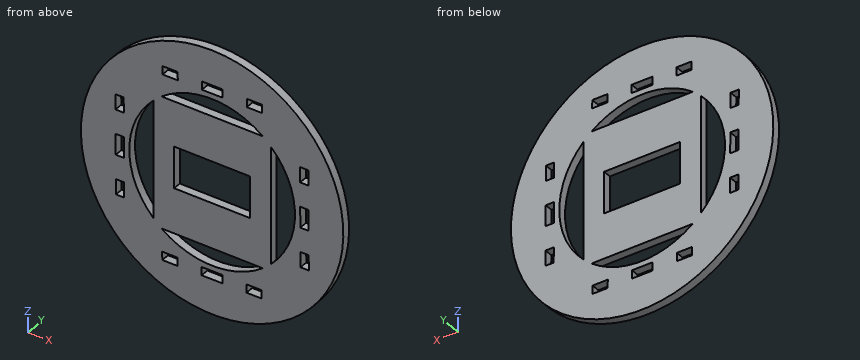
```python
from build123d import *

# Parameters (mm, degrees)
SKETCH1_R             = 95
BOSS_EXTRUDE1_DEPTH   = 6
SKETCH2_W             = 55
SKETCH2_H             = 30
CUT_EXTRUDE1_DEPTH    = 135.484199815
CAVITY1_START         = -69.821849164
CAVITY1_OUTLINE_W     = 15
CAVITY1_OUTLINE_H     = 6
CAVITY1_OUTLINE_W_2   = 11
CAVITY1_DEPTH         = 6
CAVITY1_START_2       = 63.821772898
CAVITY1_2_OUTLINE_W   = 11
CAVITY1_2_OUTLINE_H   = 6
CAVITY1_2_OUTLINE_W_2 = 15
CAVITY1_2_DEPTH       = 6
CAVITY1_START_3       = -7.051829773
CAVITY1_3_OUTLINE_W   = 6
CAVITY1_3_OUTLINE_H   = 6
CAVITY1_3_DEPTH       = 14.103659546
CAVITY1_START_4       = -35.551829773
CAVITY1_4_OUTLINE_W   = 6
CAVITY1_4_OUTLINE_H   = 6
CAVITY1_4_DEPTH       = 10.103659546
CAVITY1_START_5       = 25.448170227
CAVITY1_5_OUTLINE_W   = 6
CAVITY1_5_OUTLINE_H   = 6
CAVITY1_5_DEPTH       = 10.103659546
CAVITY1_START_6       = -36.448170227
CAVITY1_6_OUTLINE_W   = 6
CAVITY1_6_OUTLINE_H   = 6
CAVITY1_6_DEPTH       = 0.896340454
CAVITY1_START_7       = -25.448170227
CAVITY1_7_OUTLINE_W   = 6
CAVITY1_7_OUTLINE_H   = 6
CAVITY1_7_DEPTH       = 0.896340454
CAVITY1_START_8       = -7.948170227
CAVITY1_8_OUTLINE_W   = 6
CAVITY1_8_OUTLINE_H   = 6
CAVITY1_8_DEPTH       = 0.896340454
CAVITY1_START_9       = 7.051829773
CAVITY1_9_OUTLINE_W   = 6
CAVITY1_9_OUTLINE_H   = 6
CAVITY1_9_DEPTH       = 0.896340454
CAVITY1_START_10      = 24.551829773
CAVITY1_10_OUTLINE_W  = 6
CAVITY1_10_OUTLINE_H  = 6
CAVITY1_10_DEPTH      = 0.896340454
CAVITY1_START_11      = 35.551829773
CAVITY1_11_OUTLINE_W  = 6
CAVITY1_11_OUTLINE_H  = 6
CAVITY1_11_DEPTH      = 0.896340454


# Read off the part's stored shape, not the designer's step: Cavity1
with BuildPart() as part:
    # Sketch1 → Boss-Extrude1 (new body)
    with BuildSketch(Plane(origin=(0, 0, 0), x_dir=(1, 0, 0), z_dir=(0, 1, 0))):
        with Locations(Location((0, 0, 0), (0, 0, 270))):
            Circle(SKETCH1_R)
        with BuildLine():
            Line((-36.657195747, -47.5), (36.657195747, -47.5))
            ThreePointArc((36.657195747, -47.5), (0, -60), (-36.657195747, -47.5))
        make_face(mode=Mode.SUBTRACT)
        with BuildLine():
            Line((-42.5, 42.352685865), (-42.5, -42.352685865))
            ThreePointArc((-42.5, -42.352685865), (-60, 0), (-42.5, 42.352685865))
        make_face(mode=Mode.SUBTRACT)
        with BuildLine():
            Line((36.657195747, 47.5), (-36.657195747, 47.5))
            ThreePointArc((-36.657195747, 47.5), (0, 60), (36.657195747, 47.5))
        make_face(mode=Mode.SUBTRACT)
        with BuildLine():
            Line((42.5, -42.352685865), (42.5, 42.352685865))
            ThreePointArc((42.5, 42.352685865), (60, 0), (42.5, -42.352685865))
        make_face(mode=Mode.SUBTRACT)
    extrude(amount=BOSS_EXTRUDE1_DEPTH)

    # Sketch2 → Cut-Extrude1 (cut, through all)
    with BuildSketch(Plane(origin=(0, 6, 0), x_dir=(1, 0, 0), z_dir=(0, 1, 0))):
        Rectangle(SKETCH2_W, SKETCH2_H)
    extrude(amount=-CUT_EXTRUDE1_DEPTH, mode=Mode.SUBTRACT)

    # Cavity1 outline → Cavity1 (cut)
    with BuildSketch(Plane(origin=(0, 0, 0), x_dir=(0.9999872892756082, 0, 0.005041952719030872), z_dir=(0.005041952719030872, 0, -0.9999872892756083)).offset(CAVITY1_START)):
        with Locations((0.448170227, -3)):
            Rectangle(CAVITY1_OUTLINE_W, CAVITY1_OUTLINE_H)
        with Locations((30.948170227, -3)):
            Rectangle(CAVITY1_OUTLINE_W_2, CAVITY1_OUTLINE_H)
        with Locations((-30.051829773, -3)):
            Rectangle(CAVITY1_OUTLINE_W_2, CAVITY1_OUTLINE_H)
    extrude(amount=CAVITY1_DEPTH, mode=Mode.SUBTRACT)

    # Cavity1 2 outline → Cavity1 2 (cut)
    with BuildSketch(Plane(origin=(0, 0, 0), x_dir=(0.9999872892756082, 0, 0.005041952719030872), z_dir=(0.005041952719030872, 0, -0.9999872892756083)).offset(CAVITY1_START_2)):
        with Locations((30.051829773, -3)):
            Rectangle(CAVITY1_2_OUTLINE_W, CAVITY1_2_OUTLINE_H)
        with Locations((-0.448170227, -3)):
            Rectangle(CAVITY1_2_OUTLINE_W_2, CAVITY1_2_OUTLINE_H)
        with Locations((-30.948170227, -3)):
            Rectangle(CAVITY1_2_OUTLINE_W, CAVITY1_2_OUTLINE_H)
    extrude(amount=CAVITY1_2_DEPTH, mode=Mode.SUBTRACT)

    # Cavity1 3 outline → Cavity1 3 (cut)
    with BuildSketch(Plane(origin=(0, 0, 0), x_dir=(0.9999872892756082, 0, 0.005041952719030872), z_dir=(0.005041952719030872, 0, -0.9999872892756083)).offset(CAVITY1_START_3)):
        with Locations((66.821849164, -3)):
            Rectangle(CAVITY1_3_OUTLINE_W, CAVITY1_3_OUTLINE_H)
        with Locations((-66.821849164, -3)):
            Rectangle(CAVITY1_3_OUTLINE_W, CAVITY1_3_OUTLINE_H)
    extrude(amount=CAVITY1_3_DEPTH, mode=Mode.SUBTRACT)

    # Cavity1 4 outline → Cavity1 4 (cut)
    with BuildSketch(Plane(origin=(0, 0, 0), x_dir=(0.9999872892756082, 0, 0.005041952719030872), z_dir=(0.005041952719030872, 0, -0.9999872892756083)).offset(CAVITY1_START_4)):
        with Locations((66.821849164, -3)):
            Rectangle(CAVITY1_4_OUTLINE_W, CAVITY1_4_OUTLINE_H)
        with Locations((-66.821849164, -3)):
            Rectangle(CAVITY1_4_OUTLINE_W, CAVITY1_4_OUTLINE_H)
    extrude(amount=CAVITY1_4_DEPTH, mode=Mode.SUBTRACT)

    # Cavity1 5 outline → Cavity1 5 (cut)
    with BuildSketch(Plane(origin=(0, 0, 0), x_dir=(0.9999872892756082, 0, 0.005041952719030872), z_dir=(0.005041952719030872, 0, -0.9999872892756083)).offset(CAVITY1_START_5)):
        with Locations((66.821849164, -3)):
            Rectangle(CAVITY1_5_OUTLINE_W, CAVITY1_5_OUTLINE_H)
        with Locations((-66.821849164, -3)):
            Rectangle(CAVITY1_5_OUTLINE_W, CAVITY1_5_OUTLINE_H)
    extrude(amount=CAVITY1_5_DEPTH, mode=Mode.SUBTRACT)

    # Cavity1 6 outline → Cavity1 6 (cut)
    with BuildSketch(Plane(origin=(0, 0, 0), x_dir=(0.9999872892756082, 0, 0.005041952719030872), z_dir=(0.005041952719030872, 0, -0.9999872892756083)).offset(CAVITY1_START_6)):
        with Locations((-66.821849164, -3)):
            Rectangle(CAVITY1_6_OUTLINE_W, CAVITY1_6_OUTLINE_H)
    extrude(amount=CAVITY1_6_DEPTH, mode=Mode.SUBTRACT)

    # Cavity1 7 outline → Cavity1 7 (cut)
    with BuildSketch(Plane(origin=(0, 0, 0), x_dir=(0.9999872892756082, 0, 0.005041952719030872), z_dir=(0.005041952719030872, 0, -0.9999872892756083)).offset(CAVITY1_START_7)):
        with Locations((66.821849164, -3)):
            Rectangle(CAVITY1_7_OUTLINE_W, CAVITY1_7_OUTLINE_H)
    extrude(amount=CAVITY1_7_DEPTH, mode=Mode.SUBTRACT)

    # Cavity1 8 outline → Cavity1 8 (cut)
    with BuildSketch(Plane(origin=(0, 0, 0), x_dir=(0.9999872892756082, 0, 0.005041952719030872), z_dir=(0.005041952719030872, 0, -0.9999872892756083)).offset(CAVITY1_START_8)):
        with Locations((-66.821849164, -3)):
            Rectangle(CAVITY1_8_OUTLINE_W, CAVITY1_8_OUTLINE_H)
    extrude(amount=CAVITY1_8_DEPTH, mode=Mode.SUBTRACT)

    # Cavity1 9 outline → Cavity1 9 (cut)
    with BuildSketch(Plane(origin=(0, 0, 0), x_dir=(0.9999872892756082, 0, 0.005041952719030872), z_dir=(0.005041952719030872, 0, -0.9999872892756083)).offset(CAVITY1_START_9)):
        with Locations((66.821849164, -3)):
            Rectangle(CAVITY1_9_OUTLINE_W, CAVITY1_9_OUTLINE_H)
    extrude(amount=CAVITY1_9_DEPTH, mode=Mode.SUBTRACT)

    # Cavity1 10 outline → Cavity1 10 (cut)
    with BuildSketch(Plane(origin=(0, 0, 0), x_dir=(0.9999872892756082, 0, 0.005041952719030872), z_dir=(0.005041952719030872, 0, -0.9999872892756083)).offset(CAVITY1_START_10)):
        with Locations((-66.821849164, -3)):
            Rectangle(CAVITY1_10_OUTLINE_W, CAVITY1_10_OUTLINE_H)
    extrude(amount=CAVITY1_10_DEPTH, mode=Mode.SUBTRACT)

    # Cavity1 11 outline → Cavity1 11 (cut)
    with BuildSketch(Plane(origin=(0, 0, 0), x_dir=(0.9999872892756082, 0, 0.005041952719030872), z_dir=(0.005041952719030872, 0, -0.9999872892756083)).offset(CAVITY1_START_11)):
        with Locations((66.821849164, -3)):
            Rectangle(CAVITY1_11_OUTLINE_W, CAVITY1_11_OUTLINE_H)
    extrude(amount=CAVITY1_11_DEPTH, mode=Mode.SUBTRACT)


solid = part.part
```
Part model, mm, in its own coordinate system. Coordinates: 2 decimals unless noted, no trailing zeros. Loops run counter-clockwise (first coordinate to the right, second up) from the corner with the lowest first, then second, coordinate; pieces in that order, holes last. Notation, with made-up numbers: (-38, 47.5) - (-7, 47.5) arc R25 ccw to (-7, 79.5) - close; hole circle Ø5 at (39.25, 78). An arc over 180 degrees is marked (long way). Write item = value, one per line. Start each with the question number.
Item 1: Cut at D-D, the plane y = 1.35. State how many separate pieces and enclosed holes the cut face has, and give its area (3 significant figures).
Item 2: Cut at A-A, the plane z = 0. Give the cut face in (x, y), and give its area (3 significant figures).
Item 3: Wall check: L1, parallel to Z at x = -67, y = 0.55; L2, parallel to X at y = 1.4, z = -38.5; L3, parallel to Z at x = -29, y = 0.5. Give the ranges that are in metal, low to high. Write a range as from..to.
Item 4: Cut at B-B, the plane x = -20.5. Give the cut face in (y, z).
Item 5: Flat gauge pins, fed straight in: pin 1 Ø3 at (y, z) = (2, -8) entering from -X; pin 2 Ø1 at (y, z) = (5.5, 69.5) entering from -X; pin 3 Ø2 at (x, y) = (18.5, 2.5) entering from +Z. Where does each tip first touch, or does it go through?
Item 6: Cut at C-C, the plane x = 49. Give the cut face in (y, z), and give its area (3 significant figures).
The answers:
q1.separate_pieces = 1
q1.enclosed_holes = 17
q1.area = 22,500 mm2
q2.outline = (-95, 0) - (-69.82, 0) - (-69.82, 6) - (-95, 6) - close; (-63.82, 0) - (-60, 0) - (-60, 6) - (-63.82, 6) - close; (-42.5, 0) - (-27.5, 0) - (-27.5, 6) - (-42.5, 6) - close; (27.5, 0) - (42.5, 0) - (42.5, 6) - (27.5, 6) - close; (60, 0) - (63.82, 0) - (63.82, 6) - (60, 6) - close; (69.82, 0) - (95, 0) - (95, 6) - (69.82, 6) - close
q2.area = 528 mm2
q3.L1 = -67.35..-35.89, -24.89..-7.39, 7.61..25.11, 36.11..67.35
q3.L2 = -86.85..-46.02, -42.5..42.5, 46.02..86.85
q3.L3 = -90.47..-69.97, -63.97..-52.53, -47.5..47.5, 52.53..63.68, 69.68..90.47
q4.outline = (0, -92.76) - (6, -92.76) - (6, -56.39) - (0, -56.39) - close; (0, -47.5) - (6, -47.5) - (6, -15) - (0, -15) - close; (0, 15) - (6, 15) - (6, 47.5) - (0, 47.5) - close; (0, 56.39) - (6, 56.39) - (6, 92.76) - (0, 92.76) - close
q5.pin_1 = -94.78
q5.pin_2 = -65.3
q5.pin_3 = 93.37
q6.outline = (0, -81.39) - (6, -81.39) - (6, -34.63) - (0, -34.63) - close; (0, 34.63) - (6, 34.63) - (6, 81.39) - (0, 81.39) - close
q6.area = 561 mm2
